Could you check a few things on this model? Use its own coordinates, in mm. A direction names the side the tool comes from. Give positions to 0.01 mm unless a question says otherwise; leave off trailing zeros. Loops run counter-clockwise (first coordinate to the right, second up) from the corner with the lowest first, then second, coordinate; pieces in that order, holes last. Notation, with made-up numbers: (61.5, 58.25) - (108.5, 58.25) arc R29 cw to (108.5, 88.25) - close; hole circle Ø4 at (-14.75, 26). An arc over 180 degrees is marked (long way). Answer in a Markdown table with one row per item. Add a question column.
```python
from build123d import *
from build123d.topology import SkipClean

# Parameters (mm, degrees)
BOSS_EXTRUDE1_DEPTH = 3
SKETCH2_W           = 2.5
SKETCH2_H           = 11
BOSS_EXTRUDE2_DEPTH = 9.1
SKETCH3_W           = 3
SKETCH3_H           = 10.936372413
BOSS_EXTRUDE3_DEPTH = 2
SKETCH4_W           = 3
SKETCH4_H           = 10.95
BOSS_EXTRUDE4_DEPTH = 2
FILLET2_R           = 1.5
FILLET3_R           = 2
SKETCH6_W           = 20
SKETCH6_H           = 31.95
BOSS_EXTRUDE5_DEPTH = 5
CUT_EXTRUDE1_REACH  = 47.155
BOSS_EXTRUDE6_START = 1
BOSS_EXTRUDE6_DEPTH = 1
CHAMFER1_SIZE       = 1
SKETCH10_W          = 15.5
SKETCH10_H          = 20
BOSS_EXTRUDE7_DEPTH = 1.75
BOSS_EXTRUDE8_DEPTH = 12
BOSS_EXTRUDE9_DEPTH = 23.35
CHAMFER3_SIZE       = 1.7121869
CHAMFER3_SIZE_2     = 2
FILLET4_R           = 1
CHAMFER4_SIZE       = 2
CUT_EXTRUDE2_DEPTH  = 41.997050199
CUT_EXTRUDE3_DEPTH  = 3.2
SKETCH15_W          = 5.2
SKETCH15_H          = 1.9
CUT_EXTRUDE4_DEPTH  = 3.2
SKETCH16_W          = 10
SKETCH16_H          = 5
CUT_EXTRUDE5_DEPTH  = 2.2


# Some blends are built 0.0001 mm under size
with BuildPart() as part:
    # Sketch1 → Boss-Extrude1 (new body)
    with BuildSketch(Plane.XY):
        Polygon((14.5, 12.675), (-14.5, 12.675), (-14.5, 10.675), (-16.5, 10.675), (-16.5, -10.675), (16.5, -10.675), (16.5, 10.675), (14.5, 10.675), align=None)
    extrude(amount=BOSS_EXTRUDE1_DEPTH)

    # Sketch2 → Boss-Extrude2 (add)
    with BuildSketch(Plane.XY.offset(3)):
        with Locations((13.25, -0.475)):
            Rectangle(SKETCH2_W, SKETCH2_H)
        Polygon((-14.5, 5.011372413), (-14.5, -5.975), (-12, -5.975), (-12, 5.012658035), align=None)
    extrude(amount=BOSS_EXTRUDE2_DEPTH)

    # Sketch3 → Boss-Extrude3 (add)
    with BuildSketch(Plane.ZY.offset(14.5)):
        with Locations((10.6, -0.456813794)):
            Rectangle(SKETCH3_W, SKETCH3_H)
    extrude(amount=BOSS_EXTRUDE3_DEPTH)

    # Sketch4 → Boss-Extrude4 (add)
    with BuildSketch(Plane(origin=(14.5, 0, 0), x_dir=(0, 0, -1), z_dir=(1, 0, 0))):
        with Locations((-10.6, -0.45)):
            Rectangle(SKETCH4_W, SKETCH4_H)
    extrude(amount=BOSS_EXTRUDE4_DEPTH)

    # Fillet2
    fillet2_edges = [part.edges().sort_by_distance(p)[0] for p in [
        (-16.5, -0.456813793, 9.1),
        (-16.5, -0.456813793, 12.1),
        (16.5, -0.45, 9.1),
        (16.5, -0.45, 12.1),
    ]]
    fillet(fillet2_edges, radius=FILLET2_R - 0.0001)  # a hair under: the kernel refuses the full size

    # Fillet3
    fillet3_edges = [part.edges().sort_by_distance(p)[0] for p in [
        (12, -0.475, 3),
        (-12, -0.481170983, 3),
    ]]
    fillet(fillet3_edges, radius=FILLET3_R)

    # Sketch6 → Boss-Extrude5 (add)
    with BuildSketch(Plane(origin=(0, 12.675, 0), x_dir=(1, 0, 0), z_dir=(0, 1, 0))):
        with Locations((0, -18.975)):
            Rectangle(SKETCH6_W, SKETCH6_H)
    extrude(amount=-BOSS_EXTRUDE5_DEPTH)

    # Sketch7 → Cut-Extrude1 (cut, up to next)
    with BuildSketch(Plane(origin=(0, 12.675, 0), x_dir=(1, 0, 0), z_dir=(0, 1, 0)), mode=Mode.PRIVATE) as cut_extrude1_sk1:
        with BuildLine():
            Line((-4, -34.95), (4, -34.95))
            ThreePointArc((4, -34.95), (0, -30.95), (-4, -34.95))
        make_face()
    cut_extrude1_tool1 = extrude(cut_extrude1_sk1.sketch, amount=-CUT_EXTRUDE1_REACH, mode=Mode.PRIVATE) & part.part
    add(cut_extrude1_tool1.solids().sort_by_distance((0, 12.675, 33.252347))[0], mode=Mode.SUBTRACT)

    # Sketch8 → Boss-Extrude6 (add)
    with BuildSketch(Plane(origin=(0, 12.675, 0), x_dir=(1, 0, 0), z_dir=(0, 1, 0)).offset(BOSS_EXTRUDE6_START)):
        with BuildLine():
            Line((-7.5, -34.95), (-4, -34.95))
            ThreePointArc((-4, -34.95), (0, -30.95), (4, -34.95))
            Line((4, -34.95), (7.5, -34.95))
            Line((7.5, -34.95), (7.5, -31.843398282))
            Line((7.5, -31.843398282), (3.106601718, -27.45))
            Line((3.106601718, -27.45), (-3.106601718, -27.45))
            Line((-3.106601718, -27.45), (-7.5, -31.843398282))
            Line((-7.5, -31.843398282), (-7.5, -34.95))
        make_face()
    extrude(amount=-BOSS_EXTRUDE6_DEPTH)

    # Chamfer1
    chamfer1_edges = [part.edges().sort_by_distance(p)[0] for p in [
        (-7.5, 13.675, 33.396699141),
        (-5.303300859, 13.675, 29.646699141),
        (0, 13.675, 27.45),
        (5.303300859, 13.675, 29.646699141),
        (7.5, 13.675, 33.396699141),
    ]]
    chamfer(chamfer1_edges, length=CHAMFER1_SIZE - 0.0001)  # a hair under: the kernel refuses the full size

    # Sketch10 → Boss-Extrude7 (add)
    with BuildSketch(Plane.XZ.offset(-7.675)):
        with Locations((0, 13)):
            Rectangle(SKETCH10_W, SKETCH10_H)
    extrude(amount=BOSS_EXTRUDE7_DEPTH)

    # Sketch11 → Boss-Extrude8 (add)
    with BuildSketch(Plane.XY.offset(3)):
        Polygon((-7.75, 1.425), (-7.75, -2.075), (7.75, -2.075), (7.75, 1.425), (7.75, 2.925), (-7.75, 2.925), align=None)
    extrude(amount=BOSS_EXTRUDE8_DEPTH)

    # Sketch12 → Boss-Extrude9 (add, through all)
    with BuildSketch(Plane(origin=(0, 12.675, 0), x_dir=(1, 0, 0), z_dir=(0, 1, 0))):
        with BuildLine():
            Line((-16.5, 0), (-16.5, 2))
            ThreePointArc((-16.5, 2), (0.003271262, 0.509953036), (16.5, 2.070767971))
            Line((16.5, 2.070767971), (16.5, 0))
            Line((16.5, 0), (-16.5, 0))
        make_face()
    extrude(amount=-BOSS_EXTRUDE9_DEPTH)

    # Chamfer3
    # the kernel refuses this chamfer: 2, 1.717229303, 1.7121869 mm, written as the material it takes off along each edge
    with BuildSketch(Plane(origin=(16.5, 17.877033417, -2.070767971), x_dir=(-0.98467727082698, 0, 0.1743865600232151), z_dir=(0, -1, 0))) as chamfer3_piece_1:
        with BuildLine():
            Line((2.022860888, 0), (CHAMFER3_SIZE * 0.174386559999, -CHAMFER3_SIZE * 0.984677270689))
            Line((CHAMFER3_SIZE * 0.174386559999, -CHAMFER3_SIZE * 0.984677270689), (0, 0))
            ThreePointArc((0, 0), (1.040041486, -0.005678918), (2.022860888, 0))
        make_face()
    extrude(amount=33.754066833, mode=Mode.SUBTRACT)
    with BuildSketch(Plane(origin=(-16.5, 17.818365976, -2), x_dir=(0, 0, 1), z_dir=(0, -1, 0))) as chamfer3_piece_2:
        with BuildLine():
            Line((CHAMFER3_SIZE_2, 0), (0.296949553, -1.703050447))
            ThreePointArc((0.296949553, -1.703050447), (0.156514359, -0.873485517), (0, 0))
            Line((0, 0), (CHAMFER3_SIZE_2, 0))
        make_face()
    extrude(amount=33.636731952, mode=Mode.SUBTRACT)

    # Fillet4
    fillet4_edges = [part.edges().sort_by_distance(p)[0] for p in [
        (16.5, 10.675, 1.5),
        (16.5, -10.675, 1.320709464),
        (-16.5, -10.675, 1.5),
        (-16.5, 10.675, 1.5),
    ]]
    fillet(fillet4_edges, radius=FILLET4_R)

    # Chamfer4
    chamfer4_edges = [part.edges().sort_by_distance(p)[0] for p in [
        (-14.5, 12.675, 1.5),
        (14.5, 12.675, 1.5),
    ]]
    chamfer(chamfer4_edges, length=CHAMFER4_SIZE - 0.0001)  # a hair under: the kernel refuses the full size

    # Sketch13 → Cut-Extrude2 (cut, through all)
    with SkipClean():  # the faces are left unmerged after this step: merging them gives an invalid solid
        with BuildSketch(Plane.XY):
            with BuildLine():
                Line((12.5, 12.675), (16.5, 12.675))
                Line((16.5, 12.675), (16.5, 9.675))
                ThreePointArc((16.5, 9.675), (16.207106781, 10.382106781), (15.5, 10.675))
                Line((15.5, 10.675), (14.5, 10.675))
                Line((14.5, 10.675), (12.5, 12.675))
            make_face()
            with BuildLine():
                Line((-12.5, 12.675), (-16.5, 12.675))
                Line((-16.5, 12.675), (-16.5, 9.675))
                ThreePointArc((-16.5, 9.675), (-16.207106781, 10.382106781), (-15.5, 10.675))
                Line((-15.5, 10.675), (-14.5, 10.675))
                Line((-14.5, 10.675), (-12.5, 12.675))
            make_face()
        extrude(amount=-CUT_EXTRUDE2_DEPTH, mode=Mode.SUBTRACT)

    # Sketch14 → Cut-Extrude3 (cut)
    with SkipClean():  # the faces are left unmerged after this step: merging them gives an invalid solid
        with BuildSketch(Plane(origin=(10, 0, 0), x_dir=(0, 0, -1), z_dir=(1, 0, 0))):
            Polygon((-34.95, 10.875), (-34.95, 8.975), (-29.75, 8.975), (-29.75, 9.175), (-29.75, 10.675), (-29.75, 10.875), align=None)
        extrude(amount=-CUT_EXTRUDE3_DEPTH, mode=Mode.SUBTRACT)

    # Sketch15 → Cut-Extrude4 (cut)
    with SkipClean():  # the faces are left unmerged after this step: merging them gives an invalid solid
        with BuildSketch(Plane.ZY.offset(10)):
            with Locations((32.35, 9.925)):
                Rectangle(SKETCH15_W, SKETCH15_H)
        extrude(amount=-CUT_EXTRUDE4_DEPTH, mode=Mode.SUBTRACT)

    # Sketch16 → Cut-Extrude5 (cut)
    with SkipClean():  # the faces are left unmerged after this step: merging them gives an invalid solid
        with BuildSketch(Plane.XZ.offset(-7.675)):
            with Locations((0, 32.45)):
                Rectangle(SKETCH16_W, SKETCH16_H)
        extrude(amount=-CUT_EXTRUDE5_DEPTH, mode=Mode.SUBTRACT)


solid = part.part
```
(1) Please list where these lines run through material, in increasing order: line 1 (X direction, y = 0.25, z = 7); line 2 (X direction, y = -3.5, z = 6); line 3 (Y direction, x = 7.5, z = 13) (3 decimals).
(2) I want a section at B-B on z = 16. Please give me the cut outline in (x, y) (3 decimals), then the cut area to 3 significant figures.
(3) For pin 1 Ø1 at (y, z) = (9.5, 8.5) entering from -X; pin 2 Ø0.5 at (x, z) = (-15, 1) entering from +Y (3 decimals); pin 3 Ø2 at (y, z) = (10, 31.5) entering from +X, each with a flat end and sliding along its axis, tell me the tip position at first contact or that it passes through.
(4) I want a section at A-A on z = 6. Please give me the cut outline in (x, y) (3 decimals), then the cut area to 3 significant figures.
(5) We'd pull the mould along Y, two halves only. Please class faces 5 (the flat face through (15, -5.925, 11)), 6 (the flat face through (8, 8.975, 32)), 7 (the cylindrical face through (16.05, -0.37, 11.67)), 8 (the flat face through (-8, 10, 29.75)): pulls with the +Y half, pulls with the -Y half, needs draft (parallel to the pull), parting line crosses it, or undercut.
(6) On a 3-axis mill with a long thin cutter (end or side, diameter ignored), from which of +Z, -Z, +X, -X, +Y, -Y can I reach the whole of each face in a straight line? I mean faces 1 (the flat face through (-16.5, 0, 2)), 2 (the flat face through (0, 7, 23)), 3 (the flat face through (5, 9, 32)), 4 (the flat face through (-13, -1, 12.1)). Say none if no direction works.
Reported:
| question | item | result |
|---|---|---|
| 1 | line 1 | -14.5 to -12, -7.75 to 7.75, 12 to 14.5 |
| 1 | line 2 | -14.5 to -12, 12 to 14.5 |
| 1 | line 3 | -2.075 to 2.925, 5.925 to 12.675 |
| 2 | outline | (-10, 7.675) - (-7.75, 7.675) - (-7.75, 5.925) - (7.75, 5.925) - (7.75, 7.675) - (10, 7.675) - (10, 12.675) - (-10, 12.675) - close |
| 2 | area | 127 mm² |
| 3 | pin 1 | x = -10 |
| 3 | pin 2 | y = 10.675 |
| 3 | pin 3 | x = 10 |
| 4 | outline | (-14.5, -5.975) - (-12, -5.975) - (-12, 5.013) - (-14.5, 5.011) - close; (-10, 7.675) - (-7.75, 7.675) - (-7.75, 5.925) - (7.75, 5.925) - (7.75, 7.675) - (10, 7.675) - (10, 12.675) - (-10, 12.675) - close; (-7.75, -2.075) - (7.75, -2.075) - (7.75, 2.925) - (-7.75, 2.925) - close; (12, -5.975) - (14.5, -5.975) - (14.5, 5.025) - (12, 5.025) - close |
| 4 | area | 260 mm² |
| 5 | face 5 | pulls with the -Y half |
| 5 | face 6 | undercut |
| 5 | face 7 | needs draft |
| 5 | face 8 | undercut |
| 6 | face 1 | +Z, -Z, -X, +Y, -Y |
| 6 | face 2 | +Z, +X, -X, -Y |
| 6 | face 3 | +Z, -Y |
| 6 | face 4 | +Z, -X, +Y, -Y |
